Design review of the part shown in the three views and the two pictorial views. Dimensions are in mm from the part's minimum x, y and z. Coordinates: 2 decimals unless noted, no trailing zeros. Loops run counter-clockwise (first coordinate to the right, second up) from the corner with the lowest first, then second, coordinate; pieces in that order, holes last. Notation, with made-up numbers: M 76.5,40.5 L 95.5,40.5 A20 ccw 95.5,67.5 Z; hole C 17,30 d2. An arc over 180 degrees is marked long. Put each result on its own line as item: value. Start each with the question number.
(1) Take a section at A-A, the plane y = 120.65. Give the boundary of the cut face in (x, z) (1 decimal), then the cut area to 3 significant figures.
(2) Clearance check with a flat-ended pin moving along its axis: pin 1 (1 mm diameter, centred on x = 62, y = 37, fed in from -Z). State where the tip first meets the part, or that it passes through.
(3) Take a section at B-B, the plane y = 190.5. Give the boundary of the cut face in (x, z) (1 decimal).
(4) The part is to be moulded in two halves that separate along Y. For the marked faces 1, 2 and 3, say which applies: +Y half, -Y half, draft (parallel to the pull), parting line (faces both ways), or undercut.
(5) Take a section at D-D, the plane z = 6.5. Count the separate pieces of the cut face and the enclosed holes in it, then the cut area to 3 significant figures.
(6) For probe 1 along Y at (x, z) = (19.05, 7.25) (1 decimal); probe 2 along Y at (x, z) = (40, 9) (1 decimal); probe 3 along X at (y, z) = (13.5, 6.25), list the stretches that pass through material, from the lowest coordinate up. Write a range as [from, to].
(7) Take a section at C-C, the plane x = 57.15. Give the boundary of the cut face in (y, z) (1 decimal).
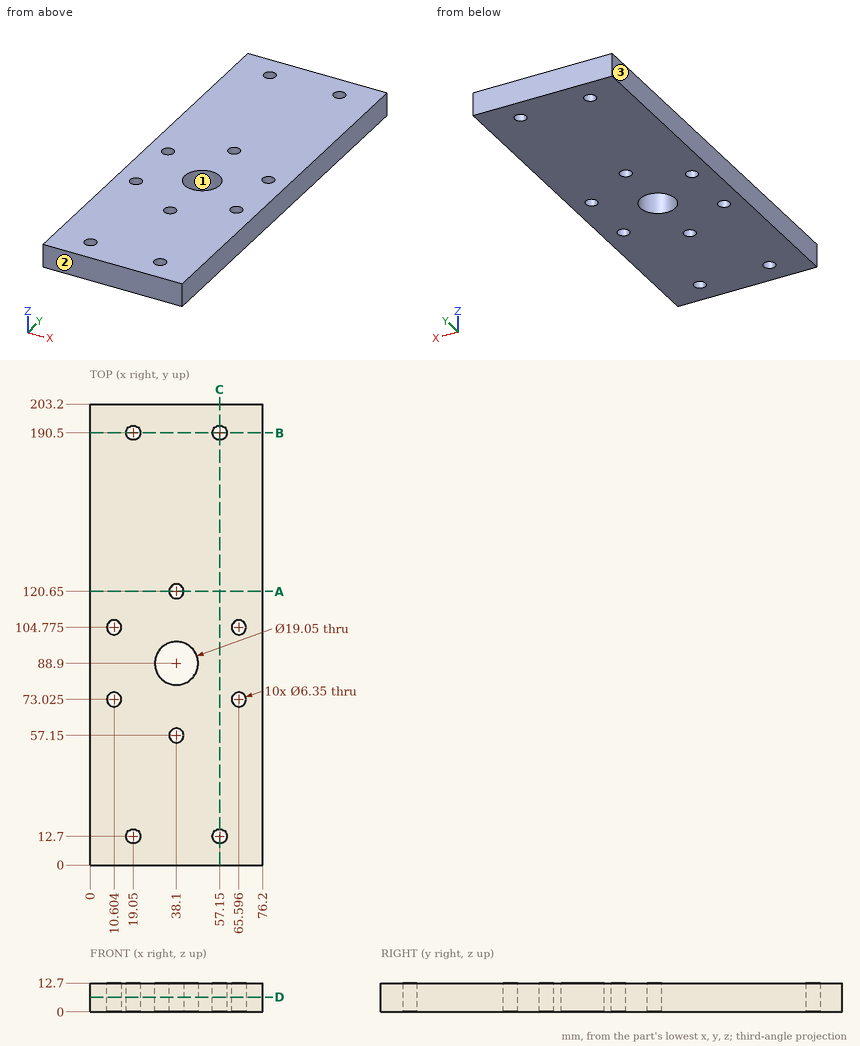
Computed values:
1. outline: M 0,0 L 34.9,0 L 34.9,12.7 L 0,12.7 Z; M 41.3,0 L 76.2,0 L 76.2,12.7 L 41.3,12.7 Z
1. area: 887 mm^2
2. pin 1: stops at z = 0
3. outline: M 0,0 L 15.9,0 L 15.9,12.7 L 0,12.7 Z; M 22.2,0 L 54,0 L 54,12.7 L 22.2,12.7 Z; M 60.3,0 L 76.2,0 L 76.2,12.7 L 60.3,12.7 Z
4. face 1: undercut
4. face 2: -Y half
4. face 3: draft
5. separate pieces: 1
5. enclosed holes: 11
5. area: 14,900 mm^2
6. probe 1: y = [0, 9.5], [15.9, 187.3], [193.7, 203.2]
6. probe 2: y = [0, 54.6], [59.7, 79.6], [98.2, 118.1], [123.2, 203.2]
6. probe 3: x = [0, 15.98], [22.12, 54.08], [60.22, 76.2]
7. outline: M 0,0 L 9.5,0 L 9.5,12.7 L 0,12.7 Z; M 15.9,0 L 187.3,0 L 187.3,12.7 L 15.9,12.7 Z; M 193.7,0 L 203.2,0 L 203.2,12.7 L 193.7,12.7 Z
